```python
from build123d import *

# Parameters (mm, degrees)
F1_DEPTH = 6


with BuildPart() as f1:
    # F0 (on Right) → F1 (new body, symmetric)
    with BuildSketch(Plane.YZ):
        Polygon((100, 90), (100, 0), (200, 0), (200, 30), (188, 30), (188, 60), (200, 60), (200, 90), align=None)
        Polygon((0, 30), (0, 0), (100, 0), (100, 90), (0, 90), (0, 60), (12, 60), (12, 30), align=None)
    extrude(amount=F1_DEPTH, both=True)


solid = f1.part
```
The model under review builds one solid part; all positions refer to its coordinate system, in mm. A direction names the side the tool comes from. Give positions to 0.01 mm unless a question says otherwise; leave off trailing zeros. Order: outer loops, then holes, each group sorted by start corner. A loop starts at its lowest first (then second) coordinate and runs counter-clockwise, first axis right, second up. Notation, with made-up numbers: (53.5, 44) - (107.5, 44) arc R34 ccw to (107.5, 80) - close; hole circle Ø11 at (11, 72). An arc over 180 degrees is marked (long way). Use CSV: the item, a comma, the result in double quotes. Start each with the question number.
Q1. We need section A-A, the plane x = 3.5. Write out the cut boundary in (y, z).
Q2. To check wall thickness, follow line 1 along Y through (x, z) = (2, 41). State the ranges of the line that lie inside material, in increasing order. Write a range as [from, to].
Q3. Tool access review of faces 1 (the flat face through (0, 0, 15)), 2 (the flat face through (0, 12, 45)), 3 (the flat face through (0, 188, 45)): name each direction out of +Z, -Z, +X, -X, +Y, -Y from which nothing blocks a thin tool from reaching the whole face with its end or side.
Q4. We need section B-B, the plane z = 49.5. Write out the cut boundary in (x, y), and give its area (3 significant figures).
Q5. Clearance check with a flat-ended pin moving along its axis: pin 1 Ø3.5 at (x, z) = (-1, 47) entering from -Y. State where the tip first meets the part, or that it passes through.
Outcome:
1,outline,"(0, 0) - (200, 0) - (200, 30) - (188, 30) - (188, 60) - (200, 60) - (200, 90) - (0, 90) - (0, 60) - (12, 60) - (12, 30) - (0, 30) - close"
2,line 1,"y = [12, 188]"
3,face 1,"+Z, -Z, +X, -X, -Y"
3,face 2,"+X, -X, -Y"
3,face 3,"+X, -X, +Y"
4,outline,"(-6, 12) - (6, 12) - (6, 188) - (-6, 188) - close"
4,area,"2,110 mm^2"
5,pin 1,"stops at y = 12"
